from build123d import *

# Parameters (mm, degrees)
F0_R     = 3.175
F1_DEPTH = 12.7
F2_R     = 6.35
F3_DEPTH = 68.1482
F5_D     = 5.5118
F5_DEPTH = 12.7
F5_TIP   = 1.65591178


with BuildPart() as f1:
    # F0 (on Front) → F1 (new body)
    with BuildSketch(Plane.XZ):
        Circle(F0_R)
    extrude(amount=F1_DEPTH)

    # F2 (on face) → F3 (join)
    with BuildSketch(Plane.XZ.offset(12.7)):
        Circle(F2_R)
    extrude(amount=F3_DEPTH)

    # F5
    with Locations(Plane.XZ.offset(80.8482)):
        with Locations((0, 0)):
            Hole(F5_D / 2, depth=F5_DEPTH)
            with Locations((0, 0, -(F5_DEPTH + F5_TIP / 2))):  # 118° drill point
                Cone(0, F5_D / 2, F5_TIP, mode=Mode.SUBTRACT)


solid = f1.part
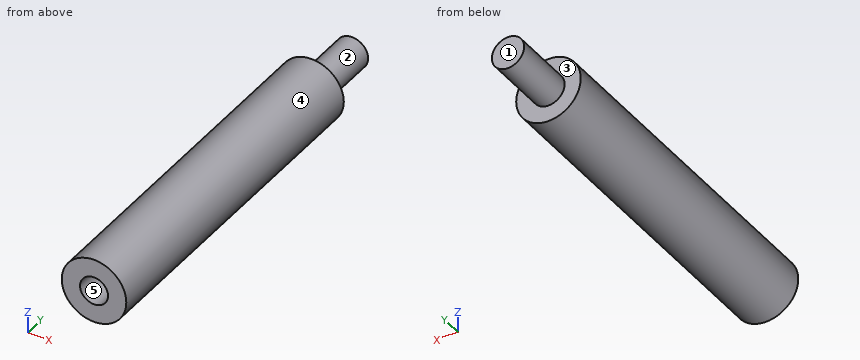
Here's how the part is built. I have some questions about the finished solid (model axes, mm). Face numbers are marked on the shaded views. A direction names the side the tool comes from. Coordinates: 2 decimals unless noted, no trailing zeros. Loops run counter-clockwise (first coordinate to the right, second up) from the corner with the lowest first, then second, coordinate; pieces in that order, holes last.
1. Imagine slicing it at D-D, the plane y = -9. Please give me the cut outline in (x, z) (3 decimals), and give its area (3 significant figures).
2. Imagine slicing it at A-A, the plane y = -18. Please give me the cut outline in (x, z), and give its area (3 significant figures).
3. If we mould it in two halves opening along Z, with no side actions, what happens to the marked faces 3, 4 and 5? For each: pulls with the +Z half, pulls with the -Z half, needs draft (parallel to the pull), parting line crosses it, or undercut.
4. I need wall thicknesses on L1, parallel to Z at x = 0, y = -71.5; L2, parallel to Y at x = 4, z = -0.25; L3, parallel to X at y = -36, z = 0.25. Which ranges of each line are inside material? Lowest first, please.
5. Imagine slicing it at B-B, the plane x = -5.25. Please give me the cut outline in (y, z).
6. Imagine slicing it at C-C, the plane z = 5.5. Please give me the cut outline in (x, y), and give its area (3 significant figures).
7. For the marked faces 1 and 2, which set-ups out of +Z, -Z, +X, -X, +Y, -Y let a thin tool reach every point of the face, with its end or its side?
8. For P1, Ø1.5, axis at y = -10, z = 1.5, coming from the +X side; P2, Ø5, axis at x = 0, z = 0, coming from the -Y side; P3, Ø6, axis at x = -3.5, y = -49, coming from the -Z side, each with a flat end and sliding along its axis, tell me the tip position at first contact or that it passes through.
Taken from the geometry:
1. outline: circle Ø6.35 at (0, 0)
1. area: 31.7 mm2
2. outline: circle Ø12.7 at (0, 0)
2. area: 127 mm2
3. face 3: needs draft
3. face 4: parting line crosses it
3. face 5: undercut
4. L1: z = -6.35 to -2.76, 2.76 to 6.35
4. L2: y = -80.85 to -12.7
4. L3: x = -6.35 to 6.35
5. outline: (-80.85, -3.57) - (-12.7, -3.57) - (-12.7, 3.57) - (-80.85, 3.57) - close
6. outline: (-3.17, -80.85) - (3.17, -80.85) - (3.17, -12.7) - (-3.17, -12.7) - close
6. area: 433 mm2
7. face 1: +Z, -Z, +X, -X, +Y
7. face 2: +Y
8. P1: stops at x = 3.09
8. P2: stops at y = -67.99
8. P3: stops at z = -6.33
